from build123d import *

# Parameters (mm, degrees)
SKETCH125_W          = 21.952
SKETCH125_H          = 70.3
SKETCH125_R          = 1.75
PAD042_DEPTH         = 4
FILLET010_R          = 2
SKETCH126_W          = 2
SKETCH126_H          = 2.1
POCKET054_DEPTH      = 35.151
POCKET054_DEPTH_BACK = 35.151
SKETCH127_R          = 3
POCKET053_DEPTH      = 2.001
SKETCH128_W          = 4.202
SKETCH128_H          = 4.8
PAD043_DEPTH         = 10
CHAMFER006_SIZE2     = 9.99
CHAMFER006_SIZE      = 1.99


with BuildPart() as part:
    # Sketch125 → Pad042 (new body)
    with BuildSketch(Plane.XY):
        with Locations((-19.024, 0)):
            Rectangle(SKETCH125_W, SKETCH125_H)
        with Locations((-14.873, 31.75)):
            Circle(SKETCH125_R, mode=Mode.SUBTRACT)
        with Locations((-14.873, -31.75)):
            Circle(SKETCH125_R, mode=Mode.SUBTRACT)
    extrude(amount=PAD042_DEPTH)

    # Fillet010
    fillet010_edges = [part.edges().sort_by_distance(p)[0] for p in [
        (-19.024, 35.15, 4),
        (-19.024, -35.15, 4),
        (-8.048, 0, 4),
        (-8.048, -35.15, 2),
        (-8.048, 35.15, 2),
    ]]
    fillet(fillet010_edges, radius=FILLET010_R)

    # Sketch126 → Pocket054 (cut, two sides)
    with BuildSketch(Plane.XZ) as pocket054_sk:
        with Locations((-29, 2.95)):
            Rectangle(SKETCH126_W, SKETCH126_H)
    extrude(amount=-POCKET054_DEPTH, mode=Mode.SUBTRACT)
    extrude(pocket054_sk.sketch, amount=POCKET054_DEPTH_BACK, mode=Mode.SUBTRACT)

    # Sketch127 → Pocket053 (cut, through all)
    with BuildSketch(Plane.XY.offset(2)):
        with Locations((-14.873, -31.75)):
            Circle(SKETCH127_R)
        with Locations((-14.873, 31.75)):
            Circle(SKETCH127_R)
    extrude(amount=POCKET053_DEPTH, mode=Mode.SUBTRACT)

    # Sketch128 → Pad043 (join)
    with BuildSketch(Plane.XY):
        with Locations((-25.899, 30.75)):
            Rectangle(SKETCH128_W, SKETCH128_H)
        with Locations((-25.899, -30.75)):
            Rectangle(SKETCH128_W, SKETCH128_H)
    extrude(amount=-PAD043_DEPTH)

    # Chamfer006
    chamfer006_edges = [part.edges().sort_by_distance(p)[0] for p in [
        (-28, 30.75, 0),
        (-28, -30.75, 0),
    ]]
    chamfer006_side = part.faces().sort_by_distance((-18.902955, 0, 0))[0]
    chamfer(chamfer006_edges, length=CHAMFER006_SIZE, length2=CHAMFER006_SIZE2, reference=chamfer006_side)


with BuildPart() as part_1:
    # Body062 placement: moved
    add(part.part.moved(Location((0, 0, 46))))


solid = part_1.part
Geometry: final body of the model. Coordinates: model frame, mm. A direction names the side the tool comes from. Round coordinates to 2 decimals unless told otherwise and drop trailing zeros. Loops run counter-clockwise (first coordinate to the right, second up) from the corner with the lowest first, then second, coordinate; pieces in that order, holes last. Notation, with made-up numbers: (58, 74.5) - (104, 74.5) arc R31 ccw to (104, 107.5) - close; hole circle Ø5 at (69, -14). An arc over 180 degrees is marked (long way). Write each question's results on one line, items separated by ' | '. Start each with the question number.
1) Line query: probe 1 along Y at (x, z) = (-26.25, 43); probe 2 along Z at (x, y) = (-13.25, 14.5); probe 3 along X at (y, z) = (-31.75, 48.8). Output: solid intervals per line, ascending. Write a range as [from, to].
2) Mould query, pull axis Y, two halves, no side actions, for faces 1 (the face through (-26, 31, 36)), 2 (the face through (-20, 35.15, 47)), 3 (the face through (-26, 28.35, 41)). Classes: released by +Y, released by -Y, zero draft, split by the parting line, or undercut.
3) Cut plane D-D on y = 19. Return loops of the section in (x, z), then the cut area to 3 significant figures.
4) Access query for faces 4 (the face through (-26, -33.15, 41)), 5 (the face through (-15.52, 28.82, 48.99)), 6 (the face through (-23.798, 31, 41)), 7 (the face through (-29, 0, 47.9)). Directions: +Z, -Z, +X, -X, +Y, -Y. A direction counts if a zero-diameter tool reaches every point of the face in a straight line with its end or side. Return the directions, or none.
5) Cut plane C-C on x = -11.25. Return loops of the section in (y, z), then the cut area to 3 significant figures.
6) First-contact query: P1, Ø5.5, axis at x = -14.873, y = -31.75, coming from the +Z side; P2, Ø2, axis at x = -13, y = 3, coming from the -Z side; P3, Ø3, axis at x = -27, z = 40.5, coming from the +Y side. Flat tips, straight axial feed; report the tip coordinate or a pass-through.
7) Cut plane B-B on z = 45.25. Return loops of the section in (x, y).
Verdict:
1) probe 1: y = [-33.15, -28.35], [28.35, 33.15] | probe 2: z = [46, 50] | probe 3: x = [-28, -17.87], [-11.87, -8.21]
2) face 1: zero draft | face 2: released by +Y | face 3: undercut
3) outline: (-30, 46) - (-8.05, 46) - (-8.05, 48) arc R2 ccw to (-10.05, 50) - (-28, 50) - (-28, 47.9) - (-30, 47.9) - close | area: 82.7 mm2
4) face 4: -Z, +X, -X, -Y | face 5: +Z | face 6: -Z, +X, +Y, -Y | face 7: +Z, -X, +Y, -Y
5) outline: (-35.15, 46) - (35.15, 46) - (35.15, 48) arc R2 ccw to (33.15, 50) - (-33.15, 50) arc R2 ccw to (-35.15, 48) - close | area: 279 mm2
6) P1: stops at z = 48 | P2: stops at z = 46 | P3: stops at y = 33.15
7) outline: (-29.84, -33.15) - (-23.8, -33.15) - (-23.8, -28.35) - (-29.84, -28.35) - close; (-29.84, 28.35) - (-23.8, 28.35) - (-23.8, 33.15) - (-29.84, 33.15) - close
